Here's the drawing with two shaded views (mm, measured from the low corner). I have some questions. A direction names the side the tool comes from. Give positions to 0.01 mm unless a question says otherwise; leave off trailing zeros. Loops run counter-clockwise (first coordinate to the right, second up) from the corner with the lowest first, then second, coordinate; pieces in that order, holes last. Notation, with made-up numbers: M 40,-1 L 71,-1 A23 cw 71,25 Z; hole C -11.5,47 d7. An arc over 180 degrees is marked long. Write item = value, one per line. Start each with the question number.
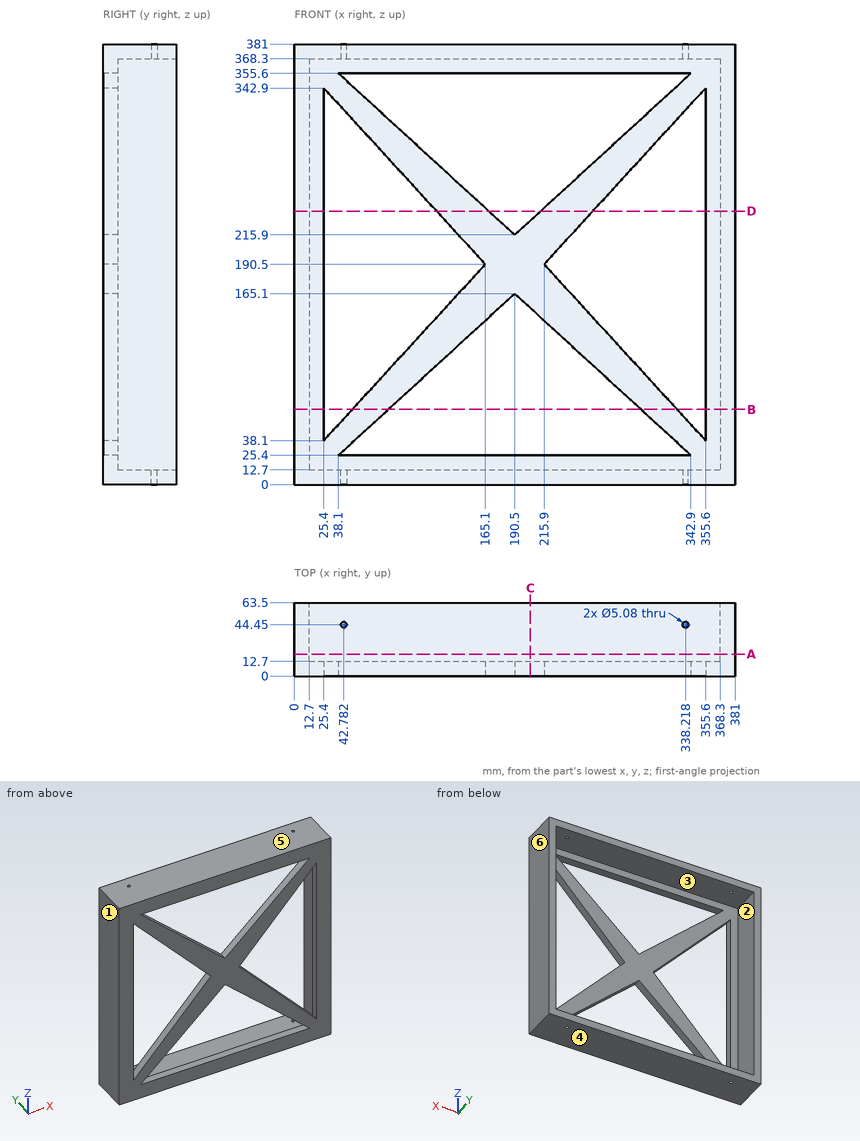
Q1. Will this pin go through, and if not, where does the flat tip stop? pin 1 (3 mm diameter, centred on x = 338.22, y = 44.45, fed in from +Z).
Q2. On a 3-axis mill with a long thin cutter (end or side, diameter ignored), from which of +Z, -Z, +X, -X, +Y, -Y can I reach the whole of each face in a straight line? I mean the marked faces 1 and 2. Say none if no direction works.
Q3. If we section it at B-B, the plane z = 65: List the corners of the cut face in (x, y) for me, then the cut area to 3 significant figures.
Q4. We'd pull the mould along Z, two halves only. Please class the marked faces 3, 4, 5 and 6: pulls with the +Z half, pulls with the -Z half, needs draft (parallel to the pull), parting line crosses it, or undercut.
Q5. If I drill on line 1 along X through (y, z) = (44, 4); line 2 along X through (y, z) = (54, 220.5), over which ranges is the centre line in solid material (lowest first)?
Q6. If we section it at A-A, the plane y = 19: List the corners of the cut face in (x, z) for me.
Q7. If we section it at C-C, the plane x = 204: List the corners of the cut face in (y, z) for me (3 decimals).
Q8. If we section it at D-D, the plane z = 236.5: List the corners of the cut face in (x, y) for me.
Resolved:
q1.pin_1 = through
q2.face_1 = +Z, -Z, -X, +Y, -Y
q2.face_2 = +Y
q3.outline = M 0,0 L 25.4,0 L 25.4,12.7 L 12.7,12.7 L 12.7,63.5 L 0,63.5 Z; M 50.06,0 L 81.3,0 L 81.3,12.7 L 50.06,12.7 Z; M 299.7,0 L 330.94,0 L 330.94,12.7 L 299.7,12.7 Z; M 355.6,0 L 381,0 L 381,63.5 L 368.3,63.5 L 368.3,12.7 L 355.6,12.7 Z
q3.area = 2,730 mm²
q4.face_3 = undercut
q4.face_4 = pulls with the -Z half
q4.face_5 = pulls with the +Z half
q4.face_6 = needs draft
q5.line_1 = 0 to 40.28, 45.28 to 335.72, 340.72 to 381
q5.line_2 = 0 to 12.7, 368.3 to 381
q6.outline = M 0,0 L 381,0 L 381,381 L 0,381 Z; hole M 12.7,12.7 L 368.3,12.7 L 368.3,368.3 L 12.7,368.3 Z
q7.outline = M 0,0 L 63.5,0 L 63.5,12.7 L 12.7,12.7 L 12.7,25.4 L 0,25.4 Z; M 0,152.725 L 12.7,152.725 L 12.7,228.275 L 0,228.275 Z; M 0,355.6 L 12.7,355.6 L 12.7,368.3 L 63.5,368.3 L 63.5,381 L 0,381 Z
q8.outline = M 0,0 L 25.4,0 L 25.4,12.7 L 12.7,12.7 L 12.7,63.5 L 0,63.5 Z; M 122.93,0 L 168.03,0 L 168.03,12.7 L 122.93,12.7 Z; M 212.97,0 L 258.07,0 L 258.07,12.7 L 212.97,12.7 Z; M 355.6,0 L 381,0 L 381,63.5 L 368.3,63.5 L 368.3,12.7 L 355.6,12.7 Z
